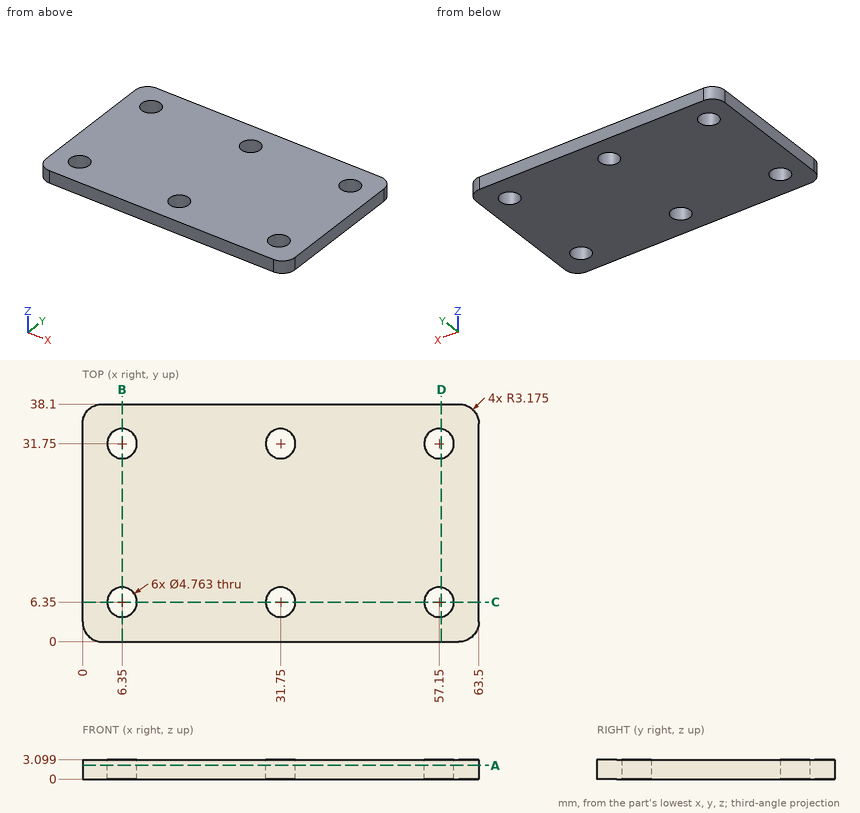
Geometry check sheet. Reference: drawing and pictorial views, mm from the part's lowest x, y, z. Round coordinates to 2 decimals unless told otherwise and drop trailing zeros. Write each loop counter-clockwise with the first axis right and the second up, starting at its lowest first coordinate (ties: lowest second). Pieces come first, ordered by that corner, then holes.
1. Section check D-D on x = 57.5. Enter the section's corners in (y, z) (1 decimal).
2. Section check C-C on y = 6.35. Enter the section's corners in (x, z).
3. Section check B-B on x = 6.35. Enter the section's corners in (y, z).
4. Scan lines: L1, parallel to Y at x = 6.35, z = 1.15; L2, parallel to Y at x = 55.5, z = 0.75 (1 decimal); L3, parallel to X at y = 30, z = 2.9 (1 decimal). Record each from-to range of solid material in increasing order.
5. Gauge pin test, flat end, axial feed: P1, Ø2, axis at x = 16, y = 27, coming from the -Z side. Record the tip position at first contact, or that the pin passes through.
6. Section check A-A on z = 2.2. State how many separate pieces and enclosed holes the cut face has, plus the area to 3 significant figures.
Answer:
1. outline: (0, 0) - (4, 0) - (4, 3.1) - (0, 3.1) - close; (8.7, 0) - (29.4, 0) - (29.4, 3.1) - (8.7, 3.1) - close; (34.1, 0) - (38.1, 0) - (38.1, 3.1) - (34.1, 3.1) - close
2. outline: (0, 0) - (3.97, 0) - (3.97, 3.1) - (0, 3.1) - close; (8.73, 0) - (29.37, 0) - (29.37, 3.1) - (8.73, 3.1) - close; (34.13, 0) - (54.77, 0) - (54.77, 3.1) - (34.13, 3.1) - close; (59.53, 0) - (63.5, 0) - (63.5, 3.1) - (59.53, 3.1) - close
3. outline: (0, 0) - (3.97, 0) - (3.97, 3.1) - (0, 3.1) - close; (8.73, 0) - (29.37, 0) - (29.37, 3.1) - (8.73, 3.1) - close; (34.13, 0) - (38.1, 0) - (38.1, 3.1) - (34.13, 3.1) - close
4. L1: y = 0 to 3.97, 8.73 to 29.37, 34.13 to 38.1
4. L2: y = 0 to 4.6, 8.1 to 30, 33.5 to 38.1
4. L3: x = 0 to 4.7, 8 to 30.1, 33.4 to 55.5, 58.8 to 63.5
5. P1: stops at z = 0
6. separate pieces: 1
6. enclosed holes: 6
6. area: 2,300 mm2
